CAD build for the part. Positions are in the model's coordinates, mm. A direction names the side the tool comes from. Coordinates: 2 decimals unless noted, no trailing zeros. Write each loop counter-clockwise with the first axis right and the second up, starting at its lowest first coordinate (ties: lowest second). Pieces come first, ordered by that corner, then holes.
```python
from build123d import *

# Parameters (mm, degrees)
ESTRUSIONE_ESTRUSIONE1_DEPTH = 5
SCHIZZO1_4_R                 = 10
ESTRUSIONE_ESTRUSIONE2_DEPTH = 6
ESTRUSIONE_ESTRUSIONE3_START = 21
ESTRUSIONE_ESTRUSIONE3_DEPTH = 27
FORO_10_0_10_1_D             = 10
FORO_10_0_10_1_CSINK_D       = 10.05
FORO_10_0_10_1_CSINK_ANGLE   = 90


with BuildPart() as part:
    # Schizzo1 → Estrusione-Estrusione1 (new, symmetric)
    with BuildSketch(Plane.XY):
        with BuildLine():
            ThreePointArc((-3.145928798, -16.706379979), (-17, 0), (-3.145928798, 16.706379979))
            Line((-3.145928798, 16.706379979), (-75, 10))
            ThreePointArc((-75, 10), (-67.928932188, 7.071067812), (-65, 0))
            ThreePointArc((-65, 0), (-67.928932188, -7.071067812), (-75, -10))
            Line((-75, -10), (-3.145928798, -16.706379979))
        make_face()
    extrude(amount=ESTRUSIONE_ESTRUSIONE1_DEPTH, both=True)

    # Schizzo1<4> → Estrusione-Estrusione2 (add, symmetric)
    with BuildSketch(Plane.XY):
        with Locations((-75, 0)):
            Circle(SCHIZZO1_4_R)
    extrude(amount=ESTRUSIONE_ESTRUSIONE2_DEPTH, both=True)

    # Schizzo1<5> → Estrusione-Estrusione3 (add)
    with BuildSketch(Plane.XY.offset(ESTRUSIONE_ESTRUSIONE3_START)):
        with BuildLine():
            ThreePointArc((17, 0), (12.02081528, 12.02081528), (0, 17))
            Line((0, 17), (-3.145928798, 16.706379979))
            ThreePointArc((-3.145928798, 16.706379979), (-17, 0), (-3.145928798, -16.706379979))
            Line((-3.145928798, -16.706379979), (0, -17))
            ThreePointArc((0, -17), (12.02081528, -12.02081528), (17, 0))
        make_face()
        with BuildLine():
            Line((-13, 3), (-9.539392014, 3))
            ThreePointArc((-9.539392014, 3), (10, 0), (-9.539392014, -3))
            Line((-9.539392014, -3), (-13, -3))
            Line((-13, -3), (-13, 3))
        make_face(mode=Mode.SUBTRACT)
    extrude(amount=-ESTRUSIONE_ESTRUSIONE3_DEPTH)

    # Foro Ø10.0 (10)-1 (through all)
    with Locations(Plane(origin=(-74.779419459, -0.265735381, 6), x_dir=(1, 0, 0), z_dir=(0, 0, 1))):
        with Locations((0, 0)):
            CounterSinkHole(FORO_10_0_10_1_D / 2, FORO_10_0_10_1_CSINK_D / 2, counter_sink_angle=FORO_10_0_10_1_CSINK_ANGLE)


solid = part.part
```
Item 1: Two-plate mould, pull along X, no slides. Class faces 6 (the flat face through (7.3, -7.3, -6)), 7 (the cylindrical face through (-69.784, -0.046, -0.096)): +X half, -X half, draft (parallel to the pull), parting line (faces both ways), or undercut.
Item 2: Which spindle directions (+Z, -Z, +X, -X, +Y, -Y) get a long thin tool onto all of the face, cutting with end or side? Do faces 1 (the cylindrical face through (-16.997, 0.33, -5.493)), 2 (the flat face through (-80, -2, -6)), 3 (the flat face through (-80, -2, 6)), 4 (the flat face through (7.3, -7.3, 21)), 5 (the flat face through (-11, 3, 8)). Say none if no direction does.
Item 3: Saw through at A-A, the plane z = 8.75. Write the cut outline in (x, y).
Item 4: Saw through at C-C, the plane y = -13. Write the cut outline in (x, z).
Item 5: Saw through at B-B, the plane y = 2. State how many separate pieces and enclosed holes the cut face has, and give its area (3 significant figures).
Item 6: Flat gauge pins, fed straight in: pin 1 Ø1.5 at (x, z) = (-65.5, -2) entering from -Y; pin 2 Ø4 at (x, z) = (-11.5, 7.5) entering from -Y; pin 3 Ø5 at (x, y) = (-22, 7.5) entering from +Z. Where does each tip first touch, or does it go through?
Item 7: Wall check: line 1 along Y through (x, z) = (0, 3.25); line 2 along X through (y, z) = (-1, 0.75); line 3 along Z through (x, y) = (-44.5, 12). Give the ranges that are in metal, low to high.
Item 8: Saw through at D-D, the plane x = -58. Write the cut outline in (y, z).
Working result:
1. face 6: draft
1. face 7: undercut
2. face 1: -Z
2. face 2: -Z, +X, -X, +Y, -Y
2. face 3: +Z, -X, +Y, -Y
2. face 4: +Z, +X, -X, +Y, -Y
2. face 5: +Z, -Z
3. outline: (-3.15, -16.71) - (0, -17) arc R17 ccw to (0, 17) - (-3.15, 16.71) arc R17 ccw to start; hole (-13, -3) - (-9.54, -3) arc R10 ccw (long way) to (-9.54, 3) - (-13, 3) - close
4. outline: (-42.86, -5) - (-10.95, -5) - (-10.95, -6) - (10.95, -6) - (10.95, 21) - (-10.95, 21) - (-10.95, 5) - (-42.86, 5) - close
5. separate pieces: 3
5. enclosed holes: 0
5. area: 907 mm2
6. pin 1: stops at y = -10.96
6. pin 2: stops at y = -14.1
6. pin 3: stops at z = 5
7. line 1: y = -17 to -10, 10 to 17
7. line 2: x = -84.95 to -79.73, -69.83 to -13, 9.95 to 16.97
7. line 3: z = -5 to 5
8. outline: (-11.59, -5) - (11.59, -5) - (11.59, 5) - (-11.59, 5) - close
